from build123d import *

# Parameters (mm, degrees)
SKETCH6_R           = 47.688639705
BOSS_EXTRUDE3_DEPTH = 25.4
BOSS_EXTRUDE4_DEPTH = 25.4
CIRPATTERN1_COUNT   = 15


with BuildPart() as part:
    # Sketch6 → Boss-Extrude3 (new body)
    with BuildSketch(Plane.XY):
        Circle(SKETCH6_R)
    extrude(amount=BOSS_EXTRUDE3_DEPTH)

    # Sketch5 → Boss-Extrude4 (add)
    with BuildSketch(Plane.XY):
        with BuildLine():
            ThreePointArc((-1.408071238, 53.84520723), (-5.630280888, 53.568544346), (-9.817746575, 52.961314735))
            add(Edge.make_bspline(
                [(-10.610061638, 46.493364569), (-10.709772142, 47.029021497), (-10.734707714, 48.102849794), (-10.568826593, 49.872777698), (-10.241208192, 51.488329618), (-9.939095864, 52.566483824), (-9.817746575, 52.961314735)],
                knots=[0, 0, 0, 0, 0.145749794, 0.286840016, 0.476245084, 0.587002811, 0.587002811, 0.587002811, 0.587002811], degree=3))
            ThreePointArc((-10.610061638, 46.493364569), (-4.984820224, 47.427396347), (0.711692296, 47.683328858))
            add(Edge.make_bspline(
                [(0.711692296, 47.683328858), (0.697854548, 48.228011376), (0.498983761, 49.283558346), (-0.031261162, 50.980320455), (-0.687612447, 52.492452993), (-1.207283759, 53.484234257), (-1.408071238, 53.84520723)],
                knots=[0, 0, 0, 0, 0.145749794, 0.286840016, 0.476245084, 0.587002811, 0.587002811, 0.587002811, 0.587002811], degree=3))
        make_face()
    boss_extrude4 = extrude(amount=BOSS_EXTRUDE4_DEPTH)

    # CirPattern1: Boss-Extrude4 ×15 about axis
    cirpattern1_axis = Axis((0, 0, 25.4), (0, 0, 1))
    for i in range(1, CIRPATTERN1_COUNT):
        add(boss_extrude4.rotate(cirpattern1_axis, i * 360 / CIRPATTERN1_COUNT))


solid = part.part
Read the model definition and answer for the solid it produces. Units are mm, in the model's axes. A direction names the side the tool comes from. Give positions to 0.01 mm unless a question says otherwise; leave off trailing zeros. Loops run counter-clockwise (first coordinate to the right, second up) from the corner with the lowest first, then second, coordinate; pieces in that order, holes last. Notation, with made-up numbers: (-12.75, -39) -> (13.25, -39) arc R32 ccw to (13.25, -5) -> close; hole circle Ø3 at (-3, 34). An arc over 180 degrees is marked (long way). Answer as CSV lines item,"result".
Item 1: For faces 1 (the face through (46.634, -9.974, 12.522)), 2 (the face through (-31.954, -35.399, 12.522)), 3 (the face through (-52.674, 11.257, 12.522)), determine the directions among +Z, -Z, +X, -X, +Y, -Y from which every point of the face is accessible in a straight line to the end or side of a thin tool.
Returned:
face 1,"+Z, -Z, +X"
face 2,"+Z, -Z"
face 3,"+Z, -Z, -X, +Y"
Item 2: Each of these flat-tipped pins is pushed along its axis until it touches: pin 1 (1.5 mm diameter, centred on x = 42, z = 2.5, fed in from -Y); pin 2 (10 mm diameter, centred on y = -15, z = 6.5, fed in from +X); pin 3 (1 mm diameter, centred on x = 11.5, z = 14.5, fed in from +Y). Where does it stop, or does it pass through?
Returned:
pin 1,"stops at y = -25.13"
pin 2,"stops at x = 50.77"
pin 3,"stops at y = 51.69"
Item 3: Determine the mould class of faces 4 (the face through (35.998, -40.068, 12.522)), 5 (the face through (-43.54, 31.71, 12.52)), 6 (the face through (38.62, 27.98, 12.52)), 7 (the face through (23.896, 41.27, 12.522)) for opening direction X: +X half, -X half, draft (parallel to the pull), parting line (faces both ways), or undercut.
Returned:
face 4,"+X half"
face 5,"-X half"
face 6,"undercut"
face 7,"undercut"
Item 4: Find section B-B on x = 5. Give the vertices of the cut face in (y, z).
Returned:
outline,"(-47.43, 0) -> (47.43, 0) -> (47.43, 25.4) -> (-47.43, 25.4) -> close"
Item 5: Find section A-A on x = -24.5. Give the vertices of the cut face in (y, z).
Returned:
outline,"(-47.97, 0) -> (47.97, 0) -> (47.97, 25.4) -> (-47.97, 25.4) -> close"
Item 6: Consider line 1 (X direction, y = -41, z = 23); line 2 (Y direction, x = -2, z = 4.5); line 3 (X direction, y = -9.5, z = 12.25). Determine where each line is inside the solid, lowest interval first. Write a range as [from, to].
Returned:
line 1,"x = [-29.83, 24.36], [29.72, 34.93]"
line 2,"y = [-53.83, 53.83]"
line 3,"x = [-53.02, 46.73]"
